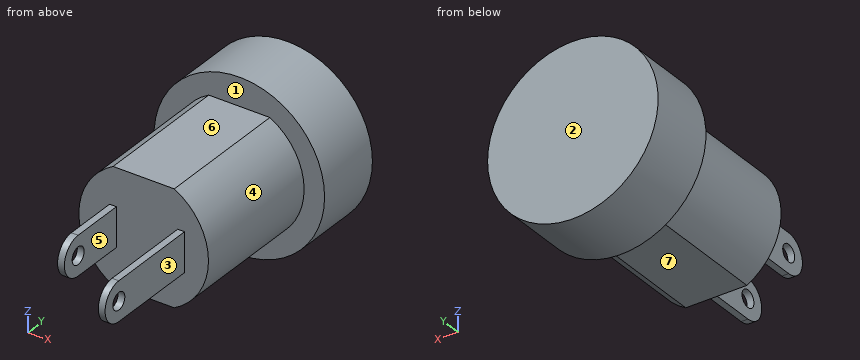
from build123d import *

# Parameters (mm, degrees)
SKETCH002_R            = 5
PAD002_DEPTH           = 4
PAD003_DEPTH           = 8
SKETCH005_R            = 0.5
PAD005_DEPTH           = 0.4
SKETCH004_R            = 0.5
PAD004_DEPTH           = 0.4
FUSION_PLACEMENT_ANGLE = 90


with BuildPart() as body001:
    # Sketch002 → Pad002 (new body)
    with BuildSketch(Plane.XY):
        Circle(SKETCH002_R)
    extrude(amount=PAD002_DEPTH)

    # Sketch003 (on Face3 of Pad002) → Pad003 (join)
    with BuildSketch(Plane.XY.offset(4)):
        with BuildLine():
            ThreePointArc((-1.793739, 3.35), (-3.8, 0), (-1.793739, -3.35))
            Line((-1.793739, -3.35), (1.793739, -3.35))
            ThreePointArc((1.793739, -3.35), (3.8, 0), (1.793739, 3.35))
            Line((-1.793739, 3.35), (1.793739, 3.35))
        make_face()
    extrude(amount=PAD003_DEPTH)


with BuildPart() as body003:
    # Sketch005 → Pad005 (new body)
    with BuildSketch(Plane.YZ):
        with BuildLine():
            Line((-1.15, 15.2), (-1.15, 12))
            Line((-1.15, 12), (1.15, 12))
            Line((1.15, 12), (1.15, 15.2))
            ThreePointArc((1.15, 15.2), (0, 16.35), (-1.15, 15.2))
        make_face()
        with Locations((0, 15.2)):
            Circle(SKETCH005_R, mode=Mode.SUBTRACT)
    extrude(amount=PAD005_DEPTH)


with BuildPart() as body003_1:
    # Body003 placement: moved
    add(body003.part.moved(Location((-2, 0, 0))))


with BuildPart() as power:
    # Sketch004 → Pad004 (new body)
    with BuildSketch(Plane.YZ):
        with BuildLine():
            Line((-1.15, 17.5), (-1.15, 12))
            Line((-1.15, 12), (1.15, 12))
            Line((1.15, 12), (1.15, 17.5))
            ThreePointArc((1.15, 17.5), (0, 18.65), (-1.15, 17.5))
        make_face()
        with Locations((0, 17.5)):
            Circle(SKETCH004_R, mode=Mode.SUBTRACT)
    extrude(amount=PAD004_DEPTH)


with BuildPart() as power_1:
    # Body002 placement: moved
    add(power.part.moved(Location((2, 0, 0))))

    # Fusion: union Body001, Body003
    add(body001.part)
    add(body003_1.part)


with BuildPart() as power_2:
    # Fusion placement: moved
    add(power_1.part.moved(Location((0, 90, 8))).rotate(Axis((0, 90, 8), (1, 0, 0)), FUSION_PLACEMENT_ANGLE))


solid = power_2.part
Geometry: final body of the model. Coordinates: model frame, mm. Face numbers are marked on the shaded views. A direction names the side the tool comes from. Coordinates: 2 decimals unless noted, no trailing zeros. Order: outer loops, then holes, each group sorted by start corner. A loop starts at its lowest first (then second) coordinate and runs counter-clockwise, first axis right, second up.
(1) Material intervals for probe 1 along Z at (x, y) = (2.15, 72.5); probe 2 along Y at (x, z) = (2.2, 8), sorted ascending.
(2) Draft query along Y for the marked faces 1, 2 and 3. Return one class per face: pulls with the +Y half, pulls with the -Y half, needs draft (parallel to the pull), parting line crosses it, or undercut.
(3) First-contact query: pin 1 (1 mm diameter, centred on y = 87.5, z = 10, fed in from +X); pin 2 (0.7 mm diameter, centred on y = 75.5, z = 8.5, fed in from -X); pin 3 (4 mm diameter, centred on x = -0.5, y = 81, fed in from -Z). Flat tips, straight axial feed; report the tip coordinate or a pass-through.
(4) Access query for the marked faces 4, 5, 6 and 7. Directions: +Z, -Z, +X, -X, +Y, -Y. A direction counts if a zero-diameter tool reaches every point of the face in a straight line with its end or side. Return the directions, or none.
(5) Section query D-D (z = 12). Return the cut outline in (x, y).
(6) Section query B-B (z = 8). Return the cut outline in (x, y), plus the area to 3 significant figures.
(7) Section query A-A (y = 76). Return the cut outline in (x, z).
(8) Section query C-C (x = 0). Return the cut outline in (y, z).
Solution:
1. probe 1: z = 6.85 to 7.5, 8.5 to 9.15
1. probe 2: y = 71.35 to 72, 73 to 90
2. face 1: pulls with the -Y half
2. face 2: pulls with the +Y half
2. face 3: needs draft
3. pin 1: stops at x = 4.77
3. pin 2: stops at x = -2
3. pin 3: stops at z = 4.65
4. face 4: +X, -Y
4. face 5: +Z, -Z, -Y
4. face 6: +Z, +X, -X, -Y
4. face 7: -Z, +X, -X, -Y
5. outline: (-3, 86) - (3, 86) - (3, 90) - (-3, 90) - close
6. outline: (-5, 86) - (-3.8, 86) - (-3.8, 78) - (-2, 78) - (-2, 75.3) - (-1.6, 75.3) - (-1.6, 78) - (2, 78) - (2, 73) - (2.4, 73) - (2.4, 78) - (3.8, 78) - (3.8, 86) - (5, 86) - (5, 90) - (-5, 90) - close; (-2, 73.65) - (-1.6, 73.65) - (-1.6, 74.3) - (-2, 74.3) - close; (2, 71.35) - (2.4, 71.35) - (2.4, 72) - (2, 72) - close
6. area: 104 mm2
7. outline: (-2, 6.85) - (-1.6, 6.85) - (-1.6, 9.15) - (-2, 9.15) - close; (2, 6.85) - (2.4, 6.85) - (2.4, 9.15) - (2, 9.15) - close
8. outline: (78, 4.65) - (86, 4.65) - (86, 3) - (90, 3) - (90, 13) - (86, 13) - (86, 11.35) - (78, 11.35) - close
